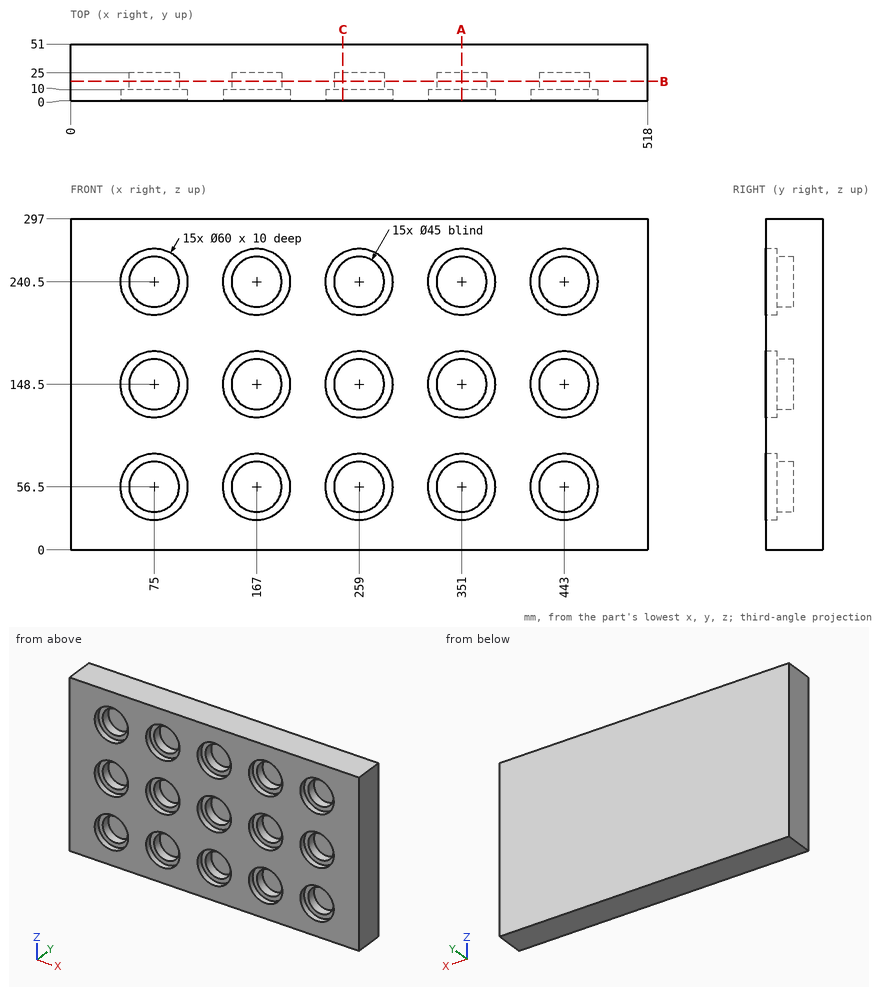
Print and shaded views of the part. All mm, measured from the part's lowest x, y and z. Give positions to 0.01 mm unless a question says otherwise; leave off trailing zeros. Loops run counter-clockwise (first coordinate to the right, second up) from the corner with the lowest first, then second, coordinate; pieces in that order, holes last. Notation, with made-up numbers: (-1.5, 49) - (33.5, 49) arc R21 ccw to (33.5, 61) - close; hole circle Ø5 at (21, -26). An arc over 180 degrees is marked (long way). One line per item, written item: value. Start each with the question number.
1. Probe L1, parallel to Z at x = 257.5, y = 19.5; L2, parallel to X at y = 4.75, z = 240.5; L3, parallel to X at y = 13, z = 56. List the from-to ranges inside material, lowest first. Write a range as from..to.
2. Slice it at C-C (x = 244.5). List the corners of the cut face in (y, z), plus the area to 3 significant figures.
3. Pin check, flat tips, straight feed: pin 1 (5 mm diameter, centred on y = 24, z = 76, fed in from -X); pin 2 (5 mm diameter, centred on x = 452.5, z = 224, fed in from -Y); pin 3 (22.5 mm diameter, centred on x = 178, z = 233, fed in from -Y). Stop position of each tip, or through.
4. Slice it at A-A (x = 351). List the corners of the cut face in (y, z), plus the area to 3 significant figures.
5. Slice it at B-B (y = 17.5). Give the number of separate pieces and of enclosed holes in the cut face, plus the area to 3 significant figures.
Solution:
1. L1: z = 0..34.05, 78.95..126.05, 170.95..218.05, 262.95..297
1. L2: x = 0..45, 105..137, 197..229, 289..321, 381..413, 473..518
1. L3: x = 0..52.51, 97.49..144.51, 189.49..236.51, 281.49..328.51, 373.49..420.51, 465.49..518
2. outline: (0, 0) - (51, 0) - (51, 297) - (0, 297) - (0, 266.76) - (10, 266.76) - (10, 257.7) - (25, 257.7) - (25, 223.3) - (10, 223.3) - (10, 214.24) - (0, 214.24) - (0, 174.76) - (10, 174.76) - (10, 165.7) - (25, 165.7) - (25, 131.3) - (10, 131.3) - (10, 122.24) - (0, 122.24) - (0, 82.76) - (10, 82.76) - (10, 73.7) - (25, 73.7) - (25, 39.3) - (10, 39.3) - (10, 30.24) - (0, 30.24) - close
2. area: 12,000 mm^2
3. pin 1: stops at x = 0
3. pin 2: stops at y = 25
3. pin 3: stops at y = 10
4. outline: (0, 0) - (51, 0) - (51, 297) - (0, 297) - (0, 270.5) - (10, 270.5) - (10, 263) - (25, 263) - (25, 218) - (10, 218) - (10, 210.5) - (0, 210.5) - (0, 178.5) - (10, 178.5) - (10, 171) - (25, 171) - (25, 126) - (10, 126) - (10, 118.5) - (0, 118.5) - (0, 86.5) - (10, 86.5) - (10, 79) - (25, 79) - (25, 34) - (10, 34) - (10, 26.5) - (0, 26.5) - close
4. area: 11,300 mm^2
5. separate pieces: 1
5. enclosed holes: 15
5. area: 130,000 mm^2
